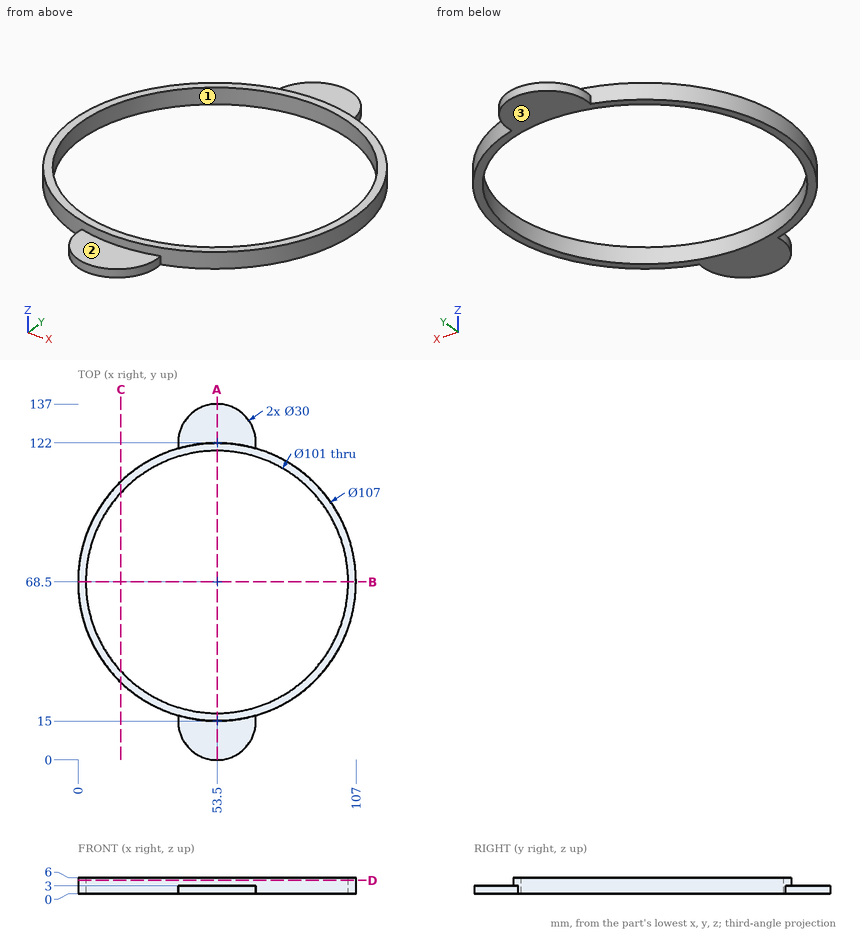
Geometry check sheet. Reference: drawing and pictorial views, mm from the part's lowest x, y, z. Round coordinates to 2 decimals unless told otherwise and drop trailing zeros. Write each loop counter-clockwise with the first axis right and the second up, starting at its lowest first coordinate (ties: lowest second). Pieces come first, ordered by that corner, then holes.
1. Section check C-C on x = 16.5. Enter the section's corners in (y, z).
2. Section check D-D on z = 5.1. Enter the section's corners in (x, y), plus the area to 3 significant figures.
3. Draft check along Z on the marked faces 1, 2 and 3. Enter one of: +Z half, -Z half, draft (parallel to the pull), parting line (faces both ways), or undercut.
4. Section check A-A on x = 53.5. Enter the section's corners in (y, z), plus the area to 3 significant figures.
5. Section check B-B on y = 68.5. Enter the section's corners in (x, z).
6. Scan lines: L1, parallel to Y at x = 53.5, z = 1.35; L2, parallel to Y at x = 53.5, z = 4.4; L3, parallel to X at y = 80, z = 1.2. Record each from-to range of solid material in increasing order.
7. Gauge pin test, flat ends, axial feed: P1, Ø8.5, axis at x = 56.5, y = 125, coming from the +Z side; P2, Ø1, axis at x = 57.5, z = 3, coming from the +Y side; P3, Ø3, axis at y = 79, z = 1, coming from the -X side; P4, Ø1, axis at y = 47, z = 2.5, coming from the +X side. Record the tip position at first contact, or that the pin passes through.
Answer:
1. outline: (29.86, 0) - (34.13, 0) - (34.13, 6) - (29.86, 6) - close; (102.87, 0) - (107.14, 0) - (107.14, 6) - (102.87, 6) - close
2. outline: circle Ø107 at (53.5, 68.5); hole circle Ø101 at (53.5, 68.5)
2. area: 980 mm2
3. face 1: draft
3. face 2: +Z half
3. face 3: -Z half
4. outline: (0, 0) - (18, 0) - (18, 6) - (15, 6) - (15, 3) - (0, 3) - close; (119, 0) - (137, 0) - (137, 3) - (122, 3) - (122, 6) - (119, 6) - close
4. area: 126 mm2
5. outline: (0, 0) - (3, 0) - (3, 6) - (0, 6) - close; (104, 0) - (107, 0) - (107, 6) - (104, 6) - close
6. L1: y = 0 to 18, 119 to 137
6. L2: y = 15 to 18, 119 to 122
6. L3: x = 1.25 to 4.33, 102.67 to 105.75
7. P1: stops at z = 6
7. P2: stops at y = 136.59
7. P3: stops at x = 0.76
7. P4: stops at x = 102.71
